Check sheet for the modelled part. Datum: model origin and axes. Units: mm. Face numbers are marked on the shaded views. A direction names the side the tool comes from. Give positions to 0.01 mm unless a question says otherwise; leave off trailing zeros. Order: outer loops, then holes, each group sorted by start corner. A loop starts at its lowest first (then second) coordinate and runs counter-clockwise, first axis right, second up. Notation, with made-up numbers: (14.25, 82) -> (67.25, 82) arc R26 ccw to (67.25, 111) -> close; hole circle Ø2 at (-28, -29.5). An arc over 180 degrees is marked (long way). Write each question's results on one line, items separated by ' | '.
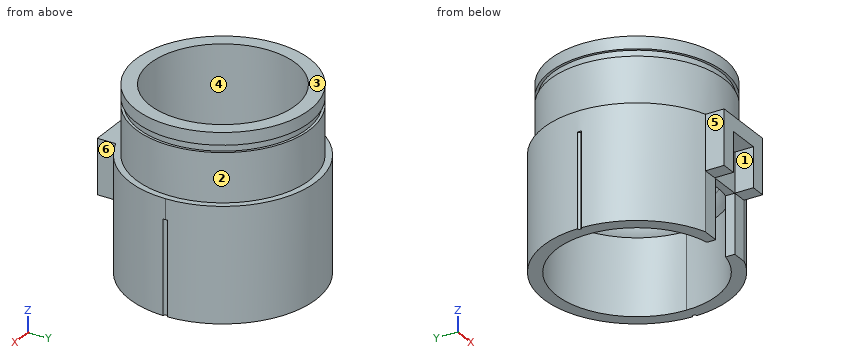
from build123d import *

# Parameters (mm, degrees)
F1_DEPTH      = 7.7216
F2_W          = 2.2098
F2_H          = 4.0132
F2_W_2        = 1.016
F2_H_2        = 2.6924
F3_DEPTH      = 1.27
F5_DEPTH      = 6.35
F6_R          = 5.9182
F6_R_2        = 4.953
F7_DEPTH      = 4.6228
F7_DEPTH_BACK = 2.54
F9_START      = -0.8382
F8_R          = 5.9182
F8_R_2        = 5.7404
F8_R_3        = 4.953
F9_DEPTH      = 0.4826
F11_W         = 2.0946894925
F11_H         = 4.0132
F12_DEPTH     = 0.6219426901


# Not quite as in the source:
# - a fillet or chamfer that OpenCascade refuses, or shapes differently, is made with other operations: its cross-section is extruded or revolved along the edge and cut away or added


with BuildPart() as f1:
    # F0 (on Top) → F1 (new body)
    with BuildSketch(Plane.XY):
        with BuildLine():
            ThreePointArc((2.1209, -5.9853390205), (0, -6.35), (-2.1209, -5.9853390205))
            Line((-2.1209, -5.9853390205), (-2.1209, -7.239))
            Line((-2.1209, -7.239), (2.1209, -7.239))
            Line((2.1209, -7.239), (2.1209, -5.9853390205))
        make_face()
        with BuildLine():
            Line((-2.1209, -5.461), (-2.1209, -5.9853390205))
            ThreePointArc((-2.1209, -5.9853390205), (0, -6.35), (2.1209, -5.9853390205))
            Line((2.1209, -5.9853390205), (2.1209, -5.461))
            Line((2.1209, -5.461), (0, -5.461))
            Line((0, -5.461), (-2.1209, -5.461))
        make_face()
        with BuildLine():
            ThreePointArc((2.1209, -5.9853390205), (5.1860493152, -3.6643406637), (6.35, 0))
            ThreePointArc((6.35, 0), (-3.6643406637, 5.1860493152), (-2.1209, -5.9853390205))
            Line((-2.1209, -5.9853390205), (-2.1209, -5.461))
            Line((-2.1209, -5.461), (0, -5.461))
            Line((0, -5.461), (2.1209, -5.461))
            Line((2.1209, -5.461), (2.1209, -5.9853390205))
        make_face()
        with BuildLine():
            ThreePointArc((5.461, 0), (3.8615101321, -3.8615101321), (0, -5.461))
            ThreePointArc((0, -5.461), (-3.8615101321, 3.8615101321), (5.461, 0))
        make_face(mode=Mode.SUBTRACT)
    extrude(amount=F1_DEPTH)

    # F2 (on face) → F3 (cut)
    with BuildSketch(Plane.XZ.offset(7.239)):
        with Locations((0, 2.0066)):
            Rectangle(F2_W, F2_H)
        with Locations((-1.6129, 2.0066)):
            Rectangle(F2_W_2, F2_H)
        with Locations((1.6129, 2.0066)):
            Rectangle(F2_W_2, F2_H)
        with Locations((0, 5.3594)):
            Rectangle(F2_W, F2_H_2)
    extrude(amount=-F3_DEPTH, mode=Mode.SUBTRACT)

    # F4 (on face) → F5 (cut)
    with BuildSketch(Plane(origin=(0, 0, 0), x_dir=(1, 0, 0), z_dir=(0, 0, -1))):
        with BuildLine():
            ThreePointArc((6.3484633, 0.1396915479), (6.2103, 0), (6.3484633, -0.1396915479))
            ThreePointArc((6.3484633, -0.1396915479), (6.35, 0), (6.3484633, 0.1396915479))
        make_face()
        with BuildLine():
            ThreePointArc((6.3484633, 0.1396915479), (6.35, 0), (6.3484633, -0.1396915479))
            ThreePointArc((6.3484633, -0.1396915479), (6.4482380095, -0.0993246369), (6.4897, 0))
            ThreePointArc((6.4897, 0), (6.4482380095, 0.0993246369), (6.3484633, 0.1396915479))
        make_face()
        with BuildLine():
            ThreePointArc((-6.3484633, -0.1396915479), (-6.2506753631, -0.0982380095), (-6.2103, 0))
            ThreePointArc((-6.2103, 0), (-6.2506753631, 0.0982380095), (-6.3484633, 0.1396915479))
            ThreePointArc((-6.3484633, 0.1396915479), (-6.35, 0), (-6.3484633, -0.1396915479))
        make_face()
        with BuildLine():
            ThreePointArc((-6.3484633, -0.1396915479), (-6.35, 0), (-6.3484633, 0.1396915479))
            ThreePointArc((-6.3484633, 0.1396915479), (-6.4897, 0), (-6.3484633, -0.1396915479))
        make_face()
    extrude(amount=-F5_DEPTH, mode=Mode.SUBTRACT)

    # F6 (on face) → F7 (join, two sides)
    with BuildSketch(Plane.XY.offset(7.7216)) as f7_sk:
        Circle(F6_R)
        Circle(F6_R_2, mode=Mode.SUBTRACT)
    extrude(amount=F7_DEPTH)
    extrude(f7_sk.sketch, amount=-F7_DEPTH_BACK)

    # F8 (on face) → F9 (cut)
    with BuildSketch(Plane.XY.offset(12.3444).offset(F9_START)):
        Circle(F8_R)
        Circle(F8_R_2, mode=Mode.SUBTRACT)
        Circle(F8_R_3)
    extrude(amount=-F9_DEPTH, mode=Mode.SUBTRACT)

    # F10: fillet of radius 1.27 on 1 edges, made by hand

    # F10_s1 → F10_t2 (revolve, cut)
    with BuildSketch(Plane.XZ):
        with BuildLine():
            ThreePointArc((5.461, 5.1816), (5.0870774674, 5.6296387337), (4.953, 6.1976))
            Line((4.953, 6.1976), (4.9276, 6.1976))
            Line((4.9276, 6.1976), (4.9276, 5.1816))
            Line((4.9276, 5.1816), (4.953, 5.1562))
            ThreePointArc((4.953, 5.1562), (5.207, 5.1562), (5.44576, 5.16128))
            Line((5.44576, 5.16128), (5.461, 5.1816))
        make_face()
    revolve(axis=Axis((0, 0, 5.1816), (0, 0, 1)), mode=Mode.SUBTRACT)

    # F11 (on face) → F12 (cut, through all)
    with BuildSketch(Plane.XZ.offset(5.969)):
        with Locations((0.0575552538, 2.0066)):
            Rectangle(F11_W, F11_H)
    extrude(amount=-F12_DEPTH, mode=Mode.SUBTRACT)


solid = f1.part
1. Gauge pin test, flat ends, axial feed: pin 1 Ø1 at (y, z) = (2, 9) entering from -X; pin 2 Ø1.4 at (y, z) = (-6.5, 6.5) entering from -X; pin 3 Ø1.6 at (x, z) = (-1, 2.5) entering from -Y. Record the tip position at first contact, or that the pin passes through.
Verdict:
pin 1: stops at x = -5.72 | pin 2: stops at x = -2.59 | pin 3: stops at y = -5.97
2. Access from +Z, -Z, +X, -X, +Y, -Y to the whole of each face (thin tool, end or side, straight path). Record for the marked faces 4, 5 and 6.
Verdict:
face 4: +Z, -Z | face 5: +Z, -Z, -X, -Y | face 6: +Z, -Z, +X, -Y
3. Material ranges on probe 1 along Y at (x, z) = (0, 8); probe 2 along Y at (x, z) = (0, 11.25); probe 3 along X at (y, z) = (3.5, 8.75), recorded low to high. Write a range as from..to.
Verdict:
probe 1: y = -5.92..-4.95, 4.95..5.92 | probe 2: y = -5.74..-4.95, 4.95..5.74 | probe 3: x = -4.77..-3.5, 3.5..4.77
4. Section check B-B on z = 9.5. Record the cut outline in (x, y), then the cut area to 3 significant figures.
Verdict:
outline: circle Ø11.84 at (0, 0); hole circle Ø9.91 at (0, 0) | area: 33.0 mm^2
5. Mould release check, pull along X, two halves, no side actions. Record for the marked faces 1, 2 and 3: +X half, -X half, draft (parallel to the pull), parting line (faces both ways), or undercut.
Verdict:
face 1: undercut | face 2: parting line | face 3: draft
